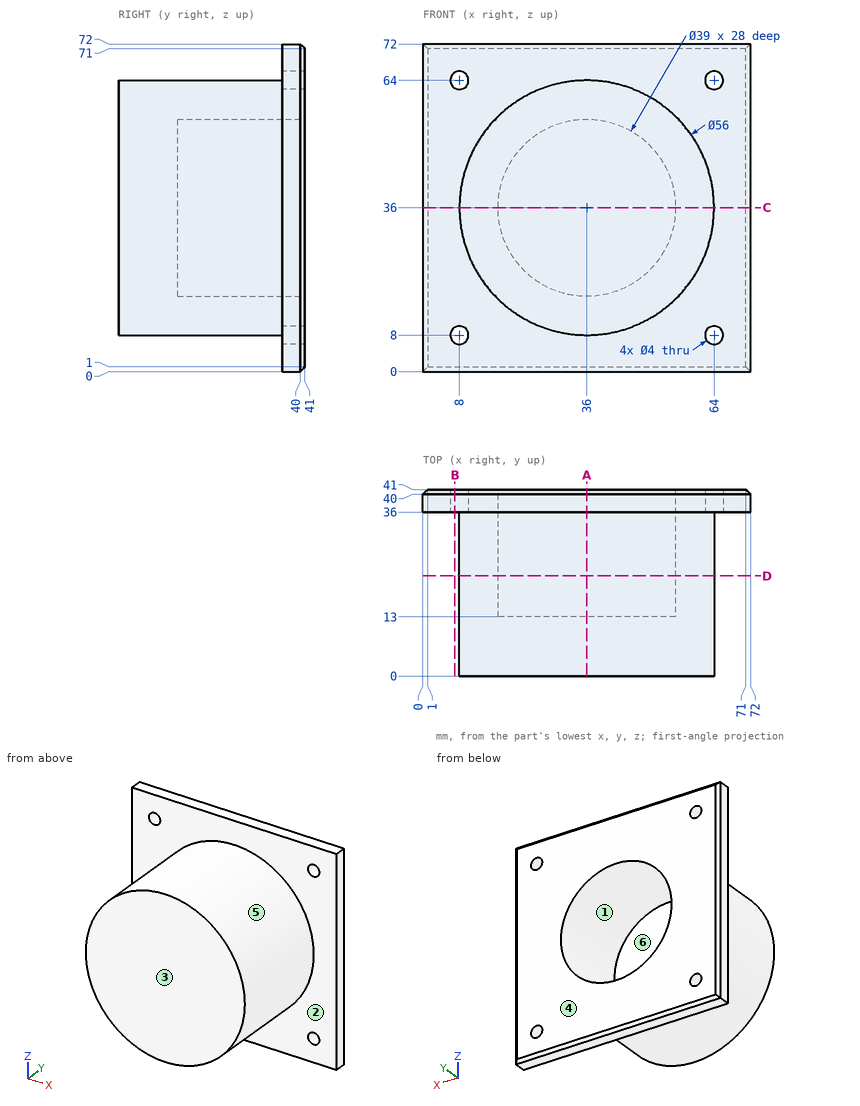
Geometry check sheet. Reference: drawing and pictorial views, mm from the part's lowest x, y, z. A direction names the side the tool comes from. Round coordinates to 2 decimals unless told otherwise and drop trailing zeros. Loops run counter-clockwise (first coordinate to the right, second up) from the corner with the lowest first, then second, coordinate; pieces in that order, holes last. Notation, with made-up numbers: (4.5, 55) - (60.5, 55) arc R14 cw to (60.5, 64) - close; hole circle Ø8 at (-37.75, -26). An arc over 180 degrees is marked (long way). Answer in a Markdown table with one row per item. Add a question column.
Q1. Section check D-D on y = 22. Enter the section's corners in (x, z).
Q2. Release check for a two-part mould opening along Z. For the marked faces 4, 5 and 6 record: pulls with the +Z half, pulls with the -Z half, needs draft (parallel to the pull), parting line crosses it, or undercut.
Q3. Gauge pin test, flat ends, axial feed: pin 1 (2 mm diameter, centred on x = 27.5, y = 26.5, fed in from -Z); pin 2 (10 mm diameter, centred on x = 56, y = 8.5, fed in from +Z); pin 3 (6.5 mm diameter, centred on x = 8, z = 8, fed in from -Y). Record the tip position at first contact, or that the pin passes through.
Q4. Tool access check on the marked faces 1, 2 and 3. Record the directions out of +Z, -Z, +X, -X, +Y, -Y that give a thin tool (end or side, any length) a straight path to the whole face; none if there is none.
Q5. Material ranges on line 1 (Z direction, x = 64, y = 38.65); line 2 (Z direction, x = 36, y = 32.75), recorded low to high.
Q6. Section check B-B on x = 7. Enter the section's corners in (y, z), plus the area to 3 significant figures.
Q7. Section check A-A on x = 36. Enter the section's corners in (y, z).
Q8. Section check C-C on z = 36. Enter the section's corners in (x, y), plus the area to 3 significant figures.
Found:
| question | item | result |
|---|---|---|
| 1 | outline | circle Ø56 at (36, 36); hole circle Ø39 at (36, 36) |
| 2 | face 4 | needs draft |
| 2 | face 5 | parting line crosses it |
| 2 | face 6 | undercut |
| 3 | pin 1 | stops at z = 9.02 |
| 3 | pin 2 | stops at z = 59.64 |
| 3 | pin 3 | stops at y = 36 |
| 4 | face 1 | +Y |
| 4 | face 2 | -Y |
| 4 | face 3 | +Z, -Z, +X, -X, -Y |
| 5 | line 1 | z = 0 to 6, 10 to 62, 66 to 72 |
| 5 | line 2 | z = 8 to 16.5, 55.5 to 64 |
| 6 | outline | (36, 0) - (40, 0) - (41, 1) - (41, 6.27) - (36, 6.27) - close; (36, 9.73) - (41, 9.73) - (41, 62.27) - (36, 62.27) - close; (36, 65.73) - (41, 65.73) - (41, 71) - (40, 72) - (36, 72) - close |
| 6 | area | 324 mm² |
| 7 | outline | (0, 8) - (36, 8) - (36, 0) - (40, 0) - (41, 1) - (41, 16.5) - (13, 16.5) - (13, 55.5) - (41, 55.5) - (41, 71) - (40, 72) - (36, 72) - (36, 64) - (0, 64) - close |
| 8 | outline | (0, 36) - (8, 36) - (8, 0) - (64, 0) - (64, 36) - (72, 36) - (72, 40) - (71, 41) - (55.5, 41) - (55.5, 13) - (16.5, 13) - (16.5, 41) - (1, 41) - (0, 40) - close |
| 8 | area | 1,280 mm² |
